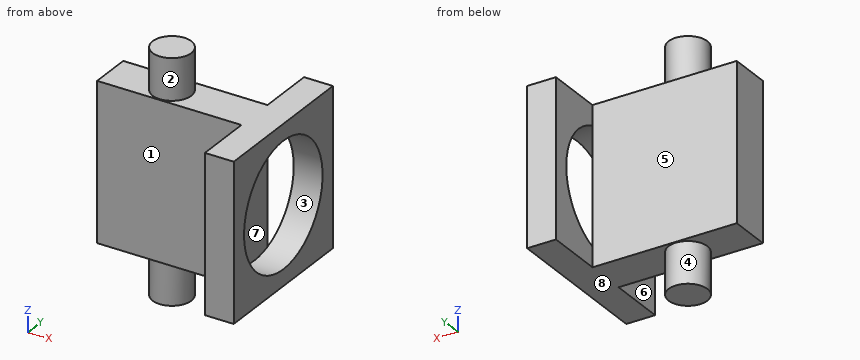
from build123d import *

# Parameters (mm, degrees)
SKETCH1_W           = 38
SKETCH1_H           = 38
SKETCH1_R           = 15.05
BOSS_EXTRUDE1_DEPTH = 7
SKETCH2_W           = 38
SKETCH2_H           = 10
BOSS_EXTRUDE2_DEPTH = 35
SKETCH3_R           = 4.7
BOSS_EXTRUDE3_DEPTH = 10


with BuildPart() as part:
    # Sketch1 → Boss-Extrude1 (new body)
    with BuildSketch(Plane(origin=(0, 0, 0), x_dir=(0, 0, -1), z_dir=(1, 0, 0))):
        Rectangle(SKETCH1_W, SKETCH1_H)
        Circle(SKETCH1_R, mode=Mode.SUBTRACT)
    extrude(amount=BOSS_EXTRUDE1_DEPTH)

    # Sketch2 → Boss-Extrude2 (add)
    with BuildSketch(Plane.ZY):
        Rectangle(SKETCH2_W, SKETCH2_H)
    extrude(amount=BOSS_EXTRUDE2_DEPTH)

    # Sketch3 → Boss-Extrude3 (add)
    with BuildSketch(Plane.XY.offset(19)):
        with Locations(Location((-20, 0, 0), (0, 0, 180))):
            Circle(SKETCH3_R)
    boss_extrude3 = extrude(amount=BOSS_EXTRUDE3_DEPTH)

    # Mirror1: Boss-Extrude3 across plane
    add(boss_extrude3.mirror(Plane.XY))


solid = part.part
Here's how the part is built. I have some questions about the finished solid (model axes, mm). Face numbers are marked on the shaded views. A direction names the side the tool comes from. Coordinates: 2 decimals unless noted, no trailing zeros. Loops run counter-clockwise (first coordinate to the right, second up) from the corner with the lowest first, then second, coordinate; pieces in that order, holes last.
1. Imagine slicing it at B-B, the plane y = 0. Please give me the cut outline in (x, z).
2. Imagine slicing it at C-C, the plane x = -20. Please give me the cut outline in (y, z).
3. For the marked faces 1, 2, 3, 4 and 5, which set-ups out of +Z, -Z, +X, -X, +Y, -Y let a thin tool reach every point of the face, with its end or its side?
4. Imagine slicing it at D-D, the plane z = 18. Please give me the cut outline in (x, y).
5. If we mould it in two halves opening along Z, with no side actions, what happens to the marked faces 6, 7 and 8? For each: pulls with the +Z half, pulls with the -Z half, needs draft (parallel to the pull), parting line crosses it, or undercut.
6. Imagine slicing it at A-A, the plane z = 0. Please give me the cut outline in (x, y), and give its area (3 significant figures).
7. I need wall thicknesses on L1, parallel to Z at x = 2.5, y = 0; L2, parallel to X at y = 17.5, z = -6.5. Which ranges of each line are inside material? Lowest first, please.
8. For P1, Ø3, axis at y = -6.5, z = -19.5, coming from the -X side; P2, Ø1, axis at x = -27, y = -0.5, coming from the -Z side; P3, Ø5, axis at x = -5.5, z = -13.5, coming from the -Y side, each with a flat end and sliding along its axis, tell me the tip position at first contact or that it passes through.
Taken from the geometry:
1. outline: (-35, -19) - (-24.7, -19) - (-24.7, -29) - (-15.3, -29) - (-15.3, -19) - (7, -19) - (7, -15.05) - (0, -15.05) - (0, 15.05) - (7, 15.05) - (7, 19) - (-15.3, 19) - (-15.3, 29) - (-24.7, 29) - (-24.7, 19) - (-35, 19) - close
2. outline: (-5, -19) - (-4.7, -19) - (-4.7, -29) - (4.7, -29) - (4.7, -19) - (5, -19) - (5, 19) - (4.7, 19) - (4.7, 29) - (-4.7, 29) - (-4.7, 19) - (-5, 19) - close
3. face 1: +Z, -Z, -X, -Y
3. face 2: +Z
3. face 3: +X
3. face 4: -Z
3. face 5: +Z, -Z, -X, +Y
4. outline: (-35, -5) - (0, -5) - (0, -19) - (7, -19) - (7, 19) - (0, 19) - (0, 5) - (-35, 5) - close
5. face 6: needs draft
5. face 7: undercut
5. face 8: pulls with the -Z half
6. outline: (-35, -5) - (0, -5) - (0, 5) - (-35, 5) - close; (0, -19) - (7, -19) - (7, -15.05) - (0, -15.05) - close; (0, 15.05) - (7, 15.05) - (7, 19) - (0, 19) - close
6. area: 405 mm2
7. L1: z = -19 to -15.05, 15.05 to 19
7. L2: x = 0 to 7
8. P1: stops at x = 0
8. P2: stops at z = -19
8. P3: stops at y = -5
